from build123d import *

# Parameters (mm, degrees)
SKETCH1_W           = 42
SKETCH1_H           = 9.5
BOSS_EXTRUDE1_DEPTH = 7.5
SKETCH2_R           = 1.55
CUT_EXTRUDE1_DEPTH  = 16
SKETCH4_R           = 3
CUT_EXTRUDE2_DEPTH  = 10.5
CHAMFER3_SIZE       = 0.5


with BuildPart() as part:
    # Sketch1 → Boss-Extrude1 (new body, symmetric)
    with BuildSketch(Plane.XY):
        Rectangle(SKETCH1_W, SKETCH1_H)
    extrude(amount=BOSS_EXTRUDE1_DEPTH, both=True)

    # Sketch2 → Cut-Extrude1 (cut, through all)
    with BuildSketch(Plane.XY.offset(7.5)):
        with Locations((-15.5, 0.75)):
            Circle(SKETCH2_R)
        with Locations((15.5, 0.75)):
            Circle(SKETCH2_R)
    extrude(amount=-CUT_EXTRUDE1_DEPTH, mode=Mode.SUBTRACT)

    # Sketch4 → Cut-Extrude2 (cut, through all)
    with BuildSketch(Plane(origin=(0, 4.75, 0), x_dir=(1, 0, 0), z_dir=(0, 1, 0))):
        with Locations((6, -2.155)):
            Circle(SKETCH4_R)
        with Locations((-6, -2.155)):
            Circle(SKETCH4_R)
    extrude(amount=-CUT_EXTRUDE2_DEPTH, mode=Mode.SUBTRACT)

    # Chamfer3
    chamfer3_edges = [part.edges().sort_by_distance(p)[0] for p in [
        (-21, 0, 7.5),
        (0, -4.75, 7.5),
        (21, 0, 7.5),
        (0, 4.75, 7.5),
        (21, -4.75, 0),
        (-21, -4.75, 0),
        (-21, 4.75, 0),
        (21, 4.75, 0),
    ]]
    chamfer(chamfer3_edges, length=CHAMFER3_SIZE)


solid = part.part
The listing builds one solid part. Answer for the finished solid, in the listing's coordinates (mm). Coordinates: 2 decimals unless noted, no trailing zeros. Write each loop counter-clockwise with the first axis right and the second up, starting at its lowest first coordinate (ties: lowest second). Pieces come first, ordered by that corner, then holes. Notation, with made-up numbers: (57.25, 28.25) - (90.25, 28.25) arc R30 cw to (90.25, 57.25) - close; hole circle Ø3 at (84.25, 80.25). An arc over 180 degrees is marked (long way). Return JSON: item names as keys, results as strings.
1. Consider line 1 along Y through (x, z) = (-15.5, 1); line 2 along Z through (x, y) = (-6, -1.5) (3 decimals). Determine where each line is inside the solid, lowest interval first.
Final values:
{"line 1": "-4.75 to -0.8, 2.3 to 4.75", "line 2": "-7.5 to -0.845, 5.155 to 7.5"}
2. The part is cut by section C-C on y = 1.5. Determine the outline of the cut face in (x, z) (3 decimals), then the cut area to 3 significant figures.
Final values:
{"outline": "(-21, -7.5) - (-16.856, -7.5) - (-16.856, 7.5) - (-20.5, 7.5) - (-21, 7) - close; (-14.144, -7.5) - (14.144, -7.5) - (14.144, 7.5) - (-14.144, 7.5) - close; (16.856, -7.5) - (21, -7.5) - (21, 7) - (20.5, 7.5) - (16.856, 7.5) - close; hole circle Ø6 at (-6, 2.155); hole circle Ø6 at (6, 2.155)", "area": "492 mm^2"}
3. This flat-tipped pin is pushed along its axis until it touches: pin 1 Ø7 at (x, z) = (-6, 2.155) entering from +Y. Where does it stop, or does it pass through?
Final values:
{"pin 1": "y = 4.75"}
4. The part is cut by section B-B on z = -4.5. Determine the outline of the cut face in (x, y), then the cut area to 3 significant figures.
Final values:
{"outline": "(-21, -4.25) - (-20.5, -4.75) - (20.5, -4.75) - (21, -4.25) - (21, 4.25) - (20.5, 4.75) - (-20.5, 4.75) - (-21, 4.25) - close; hole circle Ø3.1 at (-15.5, 0.75); hole circle Ø3.1 at (15.5, 0.75)", "area": "383 mm^2"}
5. The part is cut by section A-A on x = -6. Determine the outline of the cut face in (y, z) (3 decimals).
Final values:
{"outline": "(-4.75, -7.5) - (4.75, -7.5) - (4.75, -0.845) - (-4.75, -0.845) - close; (-4.75, 5.155) - (4.75, 5.155) - (4.75, 7) - (4.25, 7.5) - (-4.25, 7.5) - (-4.75, 7) - close"}
6. For a pull along X with two mould halves and no side action, classify faces 1 (the face through (21, 0, 0)), 2 (the face through (-17.05, 0.82, 0.11)), 3 (the face through (-21, 0, 0)), 4 (the face through (0, -4.75, 0)) as +X half, -X half, draft (parallel to the pull), parting line (faces both ways), or undercut.
Final values:
{"face 1": "+X half", "face 2": "undercut", "face 3": "-X half", "face 4": "draft"}
7. The part is cut by section D-D on x = 15.5. Determine the outline of the cut face in (y, z), then the cut area to 4 significant figures.
Final values:
{"outline": "(-4.75, -7.5) - (-0.8, -7.5) - (-0.8, 7.5) - (-4.25, 7.5) - (-4.75, 7) - close; (2.3, -7.5) - (4.75, -7.5) - (4.75, 7) - (4.25, 7.5) - (2.3, 7.5) - close", "area": "95.75 mm^2"}
